Answer from the drawing. Dimensions are ordinates in mm from the lowest x, y and z of the part. A direction names the side the tool comes from. Give positions to 0.01 mm unless a question says otherwise; leave off trailing zeros. Write each loop counter-clockwise with the first axis right and the second up, starting at its lowest first coordinate (ties: lowest second). Pieces come first, ordered by that corner, then holes. Notation, with made-up numbers: M 7,47 L 19,47 A25 cw 19,80 Z; hole C -39,12.5 d11. An arc over 180 degrees is marked long. Write each question's results on one line, items separated by ' | '. Start each with the question number.
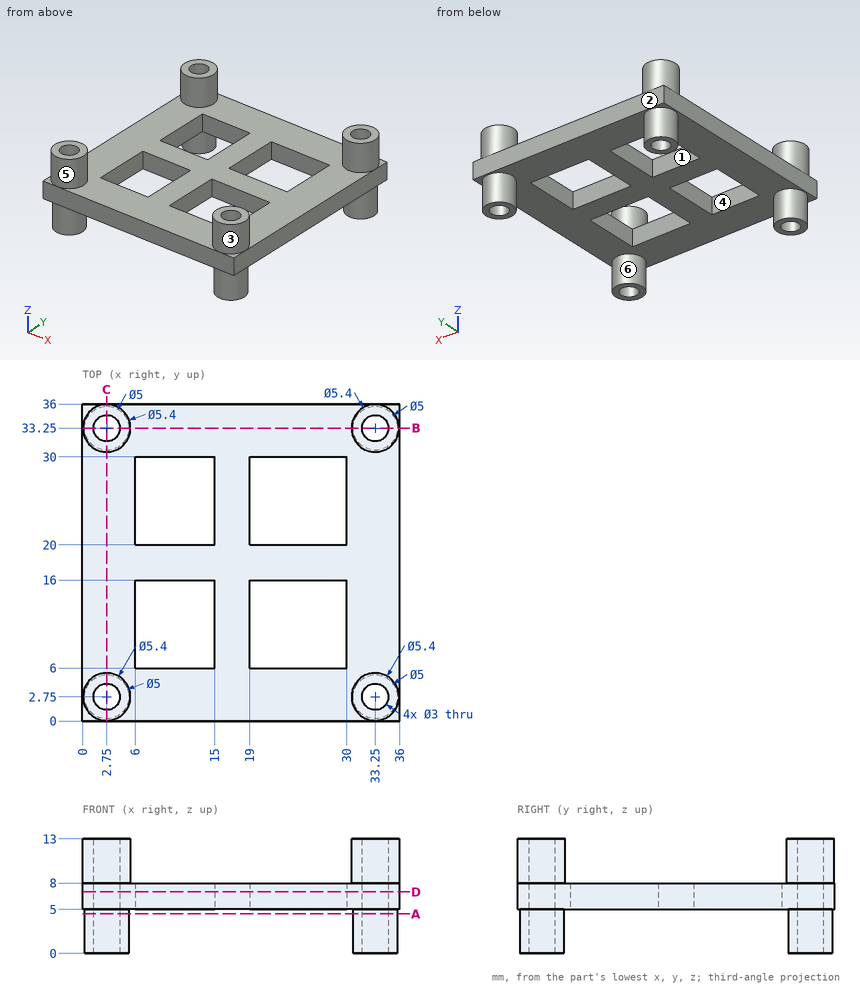
Item 1: Determine the mould class of the marked faces 1, 2 and 3 for opening direction X: +X half, -X half, draft (parallel to the pull), parting line (faces both ways), or undercut.
Item 2: Section B-B, the plane y = 33.25 is taken. Determine the outline of the cut face in (x, z).
Item 3: Given P1, Ø1.5, axis at x = 8.5, y = 18, coming from the +Z side; P2, Ø2, axis at x = 12, z = 2.5, coming from the -Y side, each flat-ended and moving along its own axis, determine where each tip first touches the part or whether it passes through.
Item 4: Straight lines are drawn through the part: line 1 (Y direction, x = 33.25, z = 4); line 2 (Y direction, x = 33.25, z = 10); line 3 (Y direction, x = 2.75, z = 7.25). For each, find the intervals that lie inside material, in ascending order.
Item 5: Section A-A, the plane z = 4.5 is taken. Determine the outline of the cut face in (x, y), then the cut area to 3 significant figures.
Item 6: For the marked faces 4, 5 and 6, determine the directions among +Z, -Z, +X, -X, +Y, -Y from which every point of the face is accessible in a straight line to the end or side of a thin tool.
Item 7: Section D-D, the plane z = 7 is taken. Give the number of separate pieces and of enclosed holes in the cut face, then the cut area to 3 significant figures.
Worked out:
1) face 1: undercut | face 2: draft | face 3: undercut
2) outline: M 0,5 L 0.25,5 L 0.25,0 L 1.25,0 L 1.25,13 L 0.05,13 L 0.05,8 L 0,8 Z; M 4.25,0 L 5.25,0 L 5.25,5 L 30.75,5 L 30.75,0 L 31.75,0 L 31.75,13 L 30.55,13 L 30.55,8 L 5.45,8 L 5.45,13 L 4.25,13 Z; M 34.75,0 L 35.75,0 L 35.75,5 L 36,5 L 36,8 L 35.95,8 L 35.95,13 L 34.75,13 Z
3) P1: stops at z = 8 | P2: passes through
4) line 1: y = 0.25 to 1.25, 4.25 to 5.25, 30.75 to 31.75, 34.75 to 35.75 | line 2: y = 0.05 to 1.25, 4.25 to 5.45, 30.55 to 31.75, 34.75 to 35.95 | line 3: y = 0 to 1.25, 4.25 to 31.75, 34.75 to 36
5) outline: C 2.75,2.75 d5; C 2.75,33.25 d5; C 33.25,2.75 d5; C 33.25,33.25 d5; hole C 2.75,2.75 d3; hole C 2.75,33.25 d3; hole C 33.25,2.75 d3; hole C 33.25,33.25 d3 | area: 50.3 mm²
6) face 4: +Z, -Z | face 5: +Z | face 6: -Z
7) separate pieces: 1 | enclosed holes: 8 | area: 868 mm²
